Check sheet for the modelled part. Datum: model origin and axes. Units: mm. A direction names the side the tool comes from. Round coordinates to 2 decimals unless told otherwise and drop trailing zeros. Order: outer loops, then holes, each group sorted by start corner. A loop starts at its lowest first (then second) coordinate and runs counter-clockwise, first axis right, second up.
```python
from build123d import *

# Parameters (mm, degrees)
SKETCH1_R               = 225
SKETCH1_R_2             = 25.4
BOSS_EXTRUDE1_DEPTH     = 20
CUT_EXTRUDE1_DEPTH      = 21
CUT_EXTRUDE1_DEPTH_BACK = 1
CUT_EXTRUDE2_START      = 20
CUT_EXTRUDE2_DEPTH      = 10


with BuildPart() as part:
    # Sketch1 → Boss-Extrude1 (new body)
    with BuildSketch(Plane(origin=(0, 0, 0), x_dir=(1, 0, 0), z_dir=(0, 1, 0))):
        Circle(SKETCH1_R)
        Circle(SKETCH1_R_2, mode=Mode.SUBTRACT)
    extrude(amount=BOSS_EXTRUDE1_DEPTH)

    # Sketch2 → Cut-Extrude1 (cut, two sides)
    with BuildSketch(Plane(origin=(0, 0, 0), x_dir=(1, 0, 0), z_dir=(0, 1, 0))) as cut_extrude1_sk:
        with BuildLine():
            Line((-178.258542487, 66.764776795), (-142.42023427, 66.764776795))
            Line((-142.42023427, 66.764776795), (-131.611855601, 0))
            Line((-131.611855601, 0), (-142.42023427, -66.764776795))
            Line((-142.42023427, -66.764776795), (-178.258542487, -66.764776795))
            add(Edge.make_bspline(
                [(-188.498059121, 0), (-188.498059121, -23.199214205), (-184.204279862, -48.203238876), (-178.258542487, -66.764776795)],
                knots=[0, 0, 0, 0, 1, 1, 1, 1], degree=3))
            add(Edge.make_bspline(
                [(-188.498059121, 0), (-188.498059121, 23.199214205), (-184.204279862, 48.203238876), (-178.258542487, 66.764776795)],
                knots=[0, 0, 0, 0, 1, 1, 1, 1], degree=3))
        make_face()
        with BuildLine():
            Line((178.258542487, -66.764776795), (142.42023427, -66.764776795))
            Line((142.42023427, -66.764776795), (131.611855601, 0))
            Line((131.611855601, 0), (142.42023427, 66.764776795))
            Line((142.42023427, 66.764776795), (178.258542487, 66.764776795))
            add(Edge.make_bspline(
                [(188.498059121, 0), (188.498059121, 23.199214205), (184.204279862, 48.203238876), (178.258542487, 66.764776795)],
                knots=[0, 0, 0, 0, 1, 1, 1, 1], degree=3))
            add(Edge.make_bspline(
                [(188.498059121, 0), (188.498059121, -23.199214205), (184.204279862, -48.203238876), (178.258542487, -66.764776795)],
                knots=[0, 0, 0, 0, 1, 1, 1, 1], degree=3))
        make_face()
    extrude(amount=CUT_EXTRUDE1_DEPTH, mode=Mode.SUBTRACT)
    extrude(cut_extrude1_sk.sketch, amount=-CUT_EXTRUDE1_DEPTH_BACK, mode=Mode.SUBTRACT)

    # Sketch3 → Cut-Extrude2 (cut)
    with BuildSketch(Plane(origin=(0, 0, 0), x_dir=(1, 0, 0), z_dir=(0, 1, 0)).offset(CUT_EXTRUDE2_START)):
        with BuildLine():
            Line((-11.5, 43.919357919), (-11.5, 194.660602074))
            ThreePointArc((-11.5, 194.660602074), (-137.885822331, 137.885822331), (-194.660602074, 11.5))
            Line((-194.660602074, 11.5), (-43.919357919, 11.5))
            ThreePointArc((-43.919357919, 11.5), (-32.102647866, 32.102647866), (-11.5, 43.919357919))
        make_face()
        with BuildLine():
            Line((11.5, 43.919357919), (11.5, 194.660602074))
            ThreePointArc((11.5, 194.660602074), (137.885822331, 137.885822331), (194.660602074, 11.5))
            Line((194.660602074, 11.5), (43.919357919, 11.5))
            ThreePointArc((43.919357919, 11.5), (32.102647866, 32.102647866), (11.5, 43.919357919))
        make_face()
        with BuildLine():
            Line((43.919357919, -11.5), (194.660602074, -11.5))
            ThreePointArc((194.660602074, -11.5), (137.885822331, -137.885822331), (11.5, -194.660602074))
            Line((11.5, -194.660602074), (11.5, -43.919357919))
            ThreePointArc((11.5, -43.919357919), (32.102647866, -32.102647866), (43.919357919, -11.5))
        make_face()
        with BuildLine():
            Line((-11.5, -43.919357919), (-11.5, -194.660602074))
            ThreePointArc((-11.5, -194.660602074), (-137.885822331, -137.885822331), (-194.660602074, -11.5))
            Line((-194.660602074, -11.5), (-43.919357919, -11.5))
            ThreePointArc((-43.919357919, -11.5), (-32.102647866, -32.102647866), (-11.5, -43.919357919))
        make_face()
    extrude(amount=-CUT_EXTRUDE2_DEPTH, mode=Mode.SUBTRACT)

    # Mirror2: part across plane


with BuildPart() as part_1:
    add(part.part)
    add(part.part.mirror(Plane.ZX))


solid = part_1.part
```
Item 1: Go/stop test with flat-tipped pins: P1, Ø8, axis at x = -71.5, y = 17, coming from the -Z side; P2, Ø11, axis at y = 15.5, z = -100.5, coming from the +X side; P3, Ø12, axis at x = 174, z = 67, coming from the -Y side. Record where each tip stops, or that it passes through.
Answer:
P1: stops at z = -214.64
P2: stops at x = 203.96
P3: stops at y = -10
Item 2: Release check for a two-part mould opening along Z. For faces 1 (the flat face through (-84, 10, -104)), 2 (the flat face through (11.5, -15, -118)) record: released by +Z, released by -Z, zero draft, split by the parting line, or undercut.
Answer:
face 1: undercut
face 2: undercut
Item 3: Sectioned sample at A-A (x = 0). Record the cut outline in (y, z), and give its area (3 significant figures).
Answer:
outline: (-20, -225) - (20, -225) - (20, -25.4) - (-20, -25.4) - close; (-20, 25.4) - (20, 25.4) - (20, 225) - (-20, 225) - close
area: 16,000 mm2
Item 4: Sectioned sample at B-B (z = 113). Record the cut outline in (x, y), and give its area (3 significant figures).
Answer:
outline: (-194.57, -20) - (-158.92, -20) - (-158.92, -10) - (-11.5, -10) - (-11.5, -20) - (11.5, -20) - (11.5, -10) - (158.92, -10) - (158.92, -20) - (194.57, -20) - (194.57, 20) - (158.92, 20) - (158.92, 10) - (11.5, 10) - (11.5, 20) - (-11.5, 20) - (-11.5, 10) - (-158.92, 10) - (-158.92, 20) - (-194.57, 20) - close
area: 9,670 mm2
Item 5: Access from +Z, -Z, +X, -X, +Y, -Y to the whole of each face (thin tool, end or side, straight path). Record for faces 3 (the flat face through (-135.74, 0.28, 25.5)), 4 (the flat face through (89, 15, -11.5)), 5 (the flat face through (-89, -15, -11.5)).
Answer:
face 3: +Y, -Y
face 4: +Y
face 5: -Y
Item 6: Sectioned sample at C-C (x = 67.5). Record the cut outline in (y, z), and give its area (3 significant figures).
Answer:
outline: (-20, -214.64) - (20, -214.64) - (20, -182.94) - (10, -182.94) - (10, -11.5) - (20, -11.5) - (20, 11.5) - (10, 11.5) - (10, 182.94) - (20, 182.94) - (20, 214.64) - (-20, 214.64) - (-20, 182.94) - (-10, 182.94) - (-10, 11.5) - (-20, 11.5) - (-20, -11.5) - (-10, -11.5) - (-10, -182.94) - (-20, -182.94) - close
area: 10,300 mm2
Item 7: Scan lines: line 1 along X through (y, z) = (7, 0); line 2 along Z through (x, y) = (0, 1); line 3 along X through (y, z) = (12.5, -120). Record each from-to range of solid material in increasing order.
Answer:
line 1: x = -225 to -188.5, -131.61 to -25.4, 25.4 to 131.61, 188.5 to 225
line 2: z = -225 to -25.4, 25.4 to 225
line 3: x = -190.33 to -153.7, -11.5 to 11.5, 153.7 to 190.33
